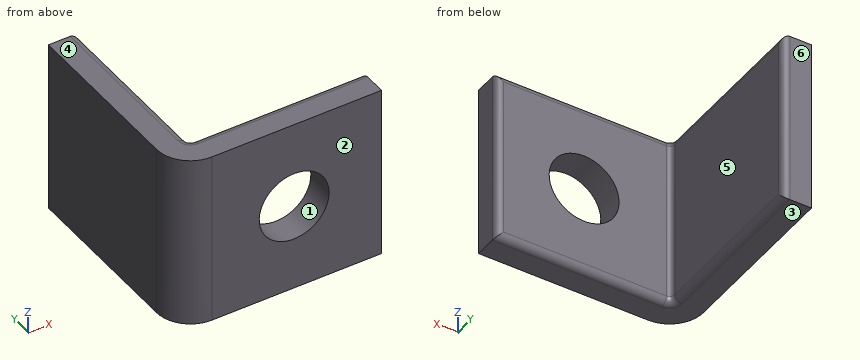
```python
from build123d import *

# Parameters (mm, degrees)
BASE_FLANGE1_DEPTH = 25
FILLET1_R          = 1
SKETCH6_R          = 5
CUT_EXTRUDE1_DEPTH = 10


# Sheet-metal steps are written as plain solids
with BuildPart() as part:
    # Sketch1 → Base-Flange1 (new body)
    with BuildSketch(Plane.XY):
        with BuildLine():
            Line((25, 0), (0.7366, 0))
            ThreePointArc((0.7366, 0), (0.215745145, 0.215745145), (0, 0.7366))
            Line((0, 0.7366), (0, 25))
            Line((0, 25), (-4.1, 25))
            Line((-4.1, 25), (-4.1, 0.7366))
            ThreePointArc((-4.1, 0.7366), (-2.683392658, -2.683392658), (0.7366, -4.1))
            Line((0.7366, -4.1), (25, -4.1))
            Line((25, -4.1), (25, 0))
        make_face()
    extrude(amount=-BASE_FLANGE1_DEPTH)

    # Fillet1
    fillet1_edges = [part.edges().sort_by_distance(p)[0] for p in [
        (0, 25, -12.5),
        (12.8683, 0, -25),
        (25, 0, -12.5),
        (0.215745145, 0.215745145, -25),
        (0, 12.8683, -25),
        (0, 12.8683, 0),
        (0.215745145, 0.215745145, 0),
        (12.8683, 0, 0),
    ]]
    fillet(fillet1_edges, radius=FILLET1_R)

    # Sketch6 → Cut-Extrude1 (cut)
    with BuildSketch(Plane(origin=(0, 0, 0), x_dir=(1, 0, 0), z_dir=(0, 1, 0))):
        with Locations(Location((12.5, 12.5, 0), (0, 0, 270))):
            Circle(SKETCH6_R)
    extrude(amount=-CUT_EXTRUDE1_DEPTH, mode=Mode.SUBTRACT)


solid = part.part
```
Here's how the part is built. I have some questions about the finished solid (model axes, mm). Face numbers are marked on the shaded views. A direction names the side the tool comes from. Round coordinates to 2 decimals unless told otherwise and drop trailing zeros. Write each loop counter-clockwise with the first axis right and the second up, starting at its lowest first coordinate (ties: lowest second). Pieces come first, ordered by that corner, then holes.
Q1. If we mould it in two halves opening along Z, with no side actions, what happens to the marked faces 1, 2, 3 and 4? For each: +Z half, -Z half, draft (parallel to the pull), parting line (faces both ways), or undercut.
Q2. If we section it at A-A on x = 12.5: Write out the boundary of the cut face in (y, z), plus the area to 3 significant figures.
Q3. Please list where these lines run through material, in increasing order: probe 1 along Y at (x, z) = (8, -21.75); probe 2 along X at (y, z) = (-1.1, -12.5).
Q4. If we section it at B-B on z = -12.5: Write out the boundary of the cut face in (x, y), plus the area to 3 significant figures.
Q5. Which directions (+Z, -Z, +X, -X, +Y, -Y) give clear straight access to the entire face, cutting with the end or side of a thin tool? Please do the marked faces 5 and 6.
Q6. Will these pins go through, and if not, where does the flat tip stop? P1, Ø3, axis at x = 9.5, y = 3, coming from the +Z side; P2, Ø12, axis at x = 12, z = -10, coming from the +Y side; P3, Ø4, axis at y = 13, z = -15.5, coming from the +X side.
Q7. If we section it at C-C on x = 5.25: Write out the boundary of the cut face in (y, z).
Q8. If we section it at D-D on z = -23.5: Write out the boundary of the cut face in (x, y).
Answer below:
1. face 1: undercut
1. face 2: draft
1. face 3: -Z half
1. face 4: +Z half
2. outline: (-4.1, -25) - (-1, -25) arc R1 ccw to (0, -24) - (0, -17.5) - (-4.1, -17.5) - close; (-4.1, -7.5) - (0, -7.5) - (0, -1) arc R1 ccw to (-1, 0) - (-4.1, 0) - close
2. area: 61.1 mm2
3. probe 1: y = -4.1 to 0
3. probe 2: x = -3.74 to 7.5, 17.5 to 25
4. outline: (-4.1, 0.74) arc R4.84 ccw to (0.74, -4.1) - (7.5, -4.1) - (7.5, 0) - (0.74, 0) arc R0.74 cw to (0, 0.74) - (0, 24) arc R1 ccw to (-1, 25) - (-4.1, 25) - close; (17.5, -4.1) - (25, -4.1) - (25, -1) arc R1 ccw to (24, 0) - (17.5, 0) - close
4. area: 175 mm2
5. face 5: +Z, -Z, +X, +Y
5. face 6: +Z, -Z, +X, -X, +Y
6. P1: passes through
6. P2: stops at y = 0
6. P3: stops at x = 0
7. outline: (-4.1, -25) - (-1, -25) arc R1 ccw to (0, -24) - (0, -1) arc R1 ccw to (-1, 0) - (-4.1, 0) - close
8. outline: (-4.1, 0.74) arc R4.84 ccw to (0.74, -4.1) - (25, -4.1) - (25, -1) arc R1 ccw to (24, 0) - (0.74, 0) arc R0.74 cw to (0, 0.74) - (0, 24) arc R1 ccw to (-1, 25) - (-4.1, 25) - close
